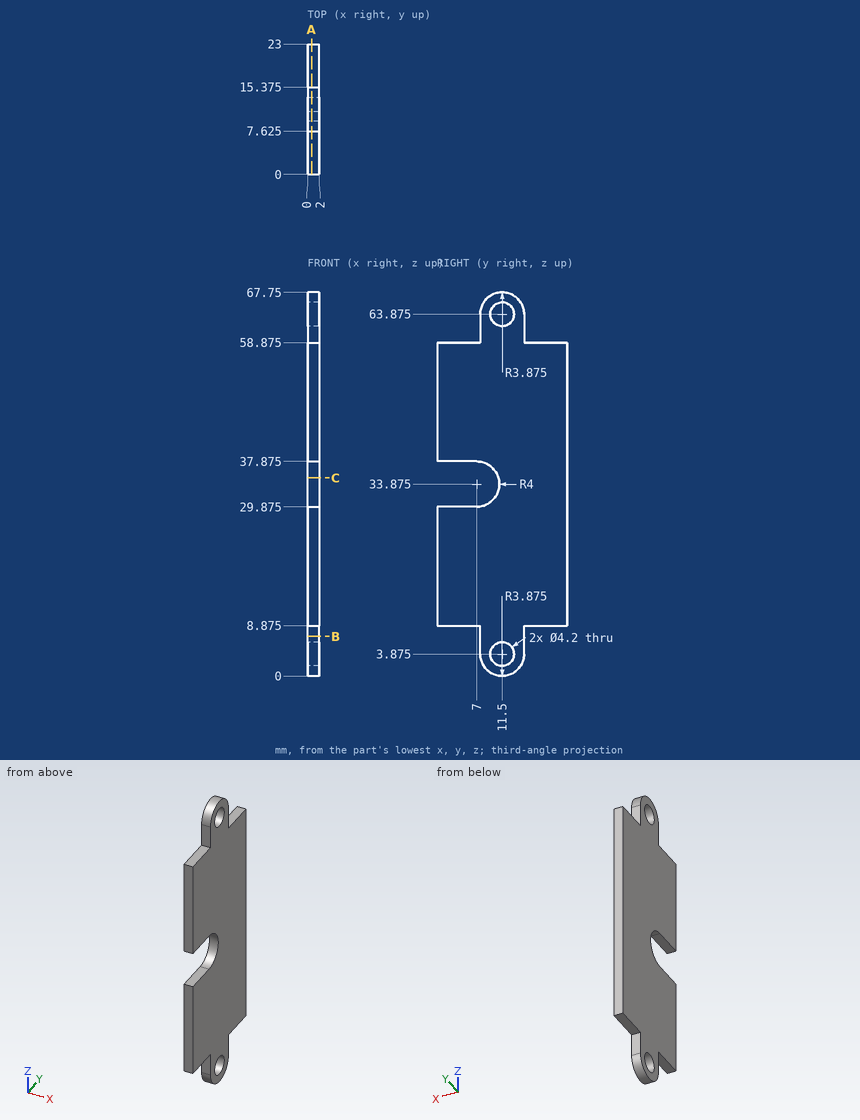
Source: three-view drawing plus pictorial views. Frame: mm from the lowest corner of the part. Coordinates: 2 decimals unless noted, no trailing zeros. Order: outer loops, then holes, each group sorted by start corner. A loop starts at its lowest first (then second) coordinate and runs counter-clockwise, first axis right, second up. Notation, with made-up numbers: (-24.75, 56) -> (-17.75, 56) arc R13 ccw to (-17.75, 78) -> close; hole circle Ø2 at (0.25, 1.5). An arc over 180 degrees is marked (long way). Write item = value, one per line.
(1) Cut plane B-B on z = 7. Return loops of the section in (x, y) (3 decimals).
Solved:
outline = (0, 7.625) -> (2, 7.625) -> (2, 15.375) -> (0, 15.375) -> close
(2) Line query: line 1 (Z direction, x = 1.35, y = 11.5) (3 decimals); line 2 (Z direction, x = 0.3, y = 6) (3 decimals); line 3 (Z direction, x = 0.7, y = 10.5). Output: solid intervals per line, ascending.
Solved:
line_1 = 0 to 1.775, 5.975 to 61.775, 65.975 to 67.75
line_2 = 8.875 to 29.875, 37.875 to 58.875
line_3 = 0.13 to 2.03, 5.72 to 31.94, 35.81 to 62.03, 65.72 to 67.62
(3) Cut plane C-C on z = 35. Return loops of the section in (x, y).
Solved:
outline = (0, 10.84) -> (2, 10.84) -> (2, 23) -> (0, 23) -> close
(4) Cut plane A-A on x = 0.7. Return loops of the section in (y, z) (3 decimals), plus the area to 3 significant figures.
Solved:
outline = (0, 8.875) -> (7.625, 8.875) -> (7.625, 3.875) arc R3.875 ccw to (15.375, 3.875) -> (15.375, 8.875) -> (23, 8.875) -> (23, 58.875) -> (15.375, 58.875) -> (15.375, 63.875) arc R3.875 ccw to (7.625, 63.875) -> (7.625, 58.875) -> (0, 58.875) -> (0, 37.875) -> (7, 37.875) arc R4 cw to (7, 29.875) -> (0, 29.875) -> close; hole circle Ø4.2 at (11.5, 3.875); hole circle Ø4.2 at (11.5, 63.875)
area = 1,170 mm²
(5) Pin query (flat end, axial travel): pin 1 Ø1 at (x, z) = (1, 62) entering from -Y (3 decimals); pin 2 Ø1 at (x, y) = (1.5, 2.5) entering from -Z (3 decimals); pin 3 Ø3.5 at (y, z) = (11.5, 63.875) entering from -X; pin 4 Ø1 at (x, y) = (1, 2) entering from +Z (3 decimals). Return the tip coordinate at first contact, or that it passes through.
Solved:
pin_1 = 7.625
pin_2 = 8.875
pin_3 = through
pin_4 = 58.875
